Autodesk Inventor part; units mm, degrees
ref_plane "YZ Plane" through (0, 0, 0) normal (1, 0, 0) x (0, 1, 0)
ref_plane "XZ Plane" through (0, 0, 0) normal (0, 1, 0) x (-1, 0, 0)
ref_plane "XY Plane" through (0, 0, 0) normal (0, 0, 1) x (1, 0, 0)
sketch "Sketch1" plane through (0, 0, 0) normal (0, 0, 1) x (1, 0, 0)
  circle A0 centre (0, 0) radius 295
  circle A1 centre (0, 0) radius 168
  dimension "d0" = 590
  dimension "d1" = 336
extrude "Extrusion1" add sketch "Sketch1" along normal blind 100
sketch "Sketch2" plane through (0, 0, 100) normal (0, 0, 1) x (1, 0, 0)
  line L0 (-204.3933, 171.1712) -> (-160.5291, 171.1712) construction
  line L1 (-160.5291, 171.1712) -> (-160.5291, 111.0696) construction
  line L2 (-160.5291, 111.0696) -> (-204.3933, 111.0696) construction
  line L3 (-204.3933, 111.0696) -> (-204.3933, 171.1712) construction
  line L4 (-245.1262, 97.2034) -> (-201.262, 97.2034) construction
  line L5 (-201.262, 97.2034) -> (-201.262, 37.1018) construction
  line L6 (-201.262, 37.1018) -> (-245.1262, 37.1018) construction
  line L7 (-245.1262, 37.1018) -> (-245.1262, 97.2034) construction
  spline S0 degree 2 poles (-185.39, 119.3884) (-190.8195, 119.3884) (-198.437, 121.6574) (-201.8001, 123.2782) knots 0 0 0 1 2 2 2
  line L8 (-201.8001, 123.2782) -> (-201.8001, 131.625)
  line L9 (-201.8001, 131.625) -> (-201.3139, 131.625)
  spline S1 degree 2 poles (-201.3139, 131.625) (-198.0319, 128.5456) (-189.7255, 125.142) (-185.8763, 125.142) knots 0 0 0 1 2 2 2
  spline S2 degree 2 poles (-185.8763, 125.142) (-180.3657, 125.142) (-174.7336, 129.7206) (-174.7336, 133.4889) knots 0 0 0 1 2 2 2
  spline S3 degree 2 poles (-174.7336, 133.4889) (-174.7336, 136.4873) (-177.6915, 140.215) (-180.8925, 141.1469) knots 0 0 0 1 2 2 2
  spline S4 degree 2 poles (-180.8925, 141.1469) (-183.202, 141.7952) (-187.0513, 142.6866) (-189.9281, 143.4159) knots 0 0 0 1 2 2 2
  spline S5 degree 2 poles (-189.9281, 143.4159) (-192.5213, 144.1048) (-196.6137, 146.1712) (-198.1939, 147.8325) knots 0 0 0 1 2 2 2
  spline S6 degree 2 poles (-198.1939, 147.8325) (-199.7336, 149.4937) (-201.4354, 153.9508) (-201.4354, 156.8681) knots 0 0 0 1 2 2 2
  spline S7 degree 2 poles (-201.4354, 156.8681) (-201.4354, 162.9459) (-191.9541, 171.1712) (-184.6202, 171.1712) knots 0 0 0 1 2 2 2
  spline S8 degree 2 poles (-184.6202, 171.1712) (-180.4062, 171.1712) (-172.9508, 169.51) (-169.7498, 167.9297) knots 0 0 0 1 2 2 2
  line L10 (-169.7498, 167.9297) -> (-169.7498, 159.9881)
  line L11 (-169.7498, 159.9881) -> (-170.2361, 159.9881)
  spline S9 degree 2 poles (-170.2361, 159.9881) (-172.6267, 162.1761) (-180.0821, 165.4176) (-184.1745, 165.4176) knots 0 0 0 1 2 2 2
  spline S10 degree 2 poles (-184.1745, 165.4176) (-188.7936, 165.4176) (-194.5067, 161.0821) (-194.5067, 157.557) knots 0 0 0 1 2 2 2
  spline S11 degree 2 poles (-194.5067, 157.557) (-194.5067, 154.3965) (-191.1437, 150.6283) (-187.9832, 149.7774) knots 0 0 0 1 2 2 2
  spline S12 degree 2 poles (-187.9832, 149.7774) (-185.8763, 149.2101) (-179.758, 147.7514) (-177.732, 147.1437) knots 0 0 0 1 2 2 2
  spline S13 degree 2 poles (-177.732, 147.1437) (-172.5862, 145.5634) (-167.805, 139.202) (-167.805, 134.5424) knots 0 0 0 1 2 2 2
  spline S14 degree 2 poles (-167.805, 134.5424) (-167.805, 131.5845) (-170.1956, 125.9119) (-172.343, 123.9265) knots 0 0 0 1 2 2 2
  spline S15 degree 2 poles (-172.343, 123.9265) (-174.7336, 121.7385) (-180.8114, 119.3884) (-185.39, 119.3884) knots 0 0 0 1 2 2 2
  spline S16 degree 2 poles (-200.6367, 72.1629) (-200.6367, 65.3152) (-206.1877, 54.2942) (-210.8474, 51.2147) knots 0 0 0 1 2 2 2
  spline S17 degree 2 poles (-210.8474, 51.2147) (-214.6561, 48.8241) (-222.4762, 47.2034) (-228.554, 47.2034) knots 0 0 0 1 2 2 2
  line L12 (-228.554, 47.2034) -> (-240.0613, 47.2034)
  line L13 (-240.0613, 47.2034) -> (-240.0613, 97.2034)
  line L14 (-240.0613, 97.2034) -> (-228.6756, 97.2034)
  spline S18 degree 2 poles (-228.6756, 97.2034) (-221.6253, 97.2034) (-213.6027, 95.0964) (-210.7663, 93.2326) knots 0 0 0 1 2 2 2
  spline S19 degree 2 poles (-210.7663, 93.2326) (-205.9446, 90.0316) (-200.6367, 79.4562) (-200.6367, 72.1629) knots 0 0 0 1 2 2 2
  spline S20 degree 2 poles (-207.5654, 72.2439) (-207.5654, 77.9976) (-211.3741, 86.1418) (-215.1424, 88.4514) knots 0 0 0 1 2 2 2
  spline S21 degree 2 poles (-215.1424, 88.4514) (-217.8166, 90.0316) (-223.8539, 91.4498) (-228.3514, 91.4498) knots 0 0 0 1 2 2 2
  line L15 (-228.3514, 91.4498) -> (-233.4163, 91.4498)
  line L16 (-233.4163, 91.4498) -> (-233.4163, 52.957)
  line L17 (-233.4163, 52.957) -> (-228.3514, 52.957)
  spline S22 degree 2 poles (-228.3514, 52.957) (-223.9349, 52.957) (-217.2493, 54.3752) (-214.5346, 56.2796) knots 0 0 0 1 2 2 2
  spline S23 degree 2 poles (-214.5346, 56.2796) (-211.05, 58.6297) (-207.5654, 66.4092) (-207.5654, 72.2439) knots 0 0 0 1 2 2 2
  point P0 (0, 0)
extrude "Extrusion2" add sketch "Sketch2" along normal blind 20
sketch "Sketch3" plane through (0, 0, 100) normal (0, 0, 1) x (1, 0, 0)
  circle A0 centre (-107.4544, 206.725) radius 38.7006
  line L0 (0, 260.9541) -> (30, 208.9926)
  line L1 (0, 260.9541) -> (60, 260.9541) construction
  line L2 (30, 208.9926) -> (-30, 208.9926)
  line L3 (-30, 208.9926) -> (0, 260.9541)
  line L4 (74.2712, 223.542) -> (129.0294, 200.0839)
  line L5 (129.0294, 200.0839) -> (129.6987, 201.6462)
  line L6 (129.6987, 201.6462) -> (74.9405, 225.1043)
  line L7 (74.9405, 225.1043) -> (74.2712, 223.542)
  line L8 (74.2712, 223.542) -> (129.6987, 201.6462) construction
  line L9 (129.0294, 200.0839) -> (74.9405, 225.1043) construction
  line L10 (63.2876, 195.758) -> (118.0458, 172.2999)
  line L11 (118.0458, 172.2999) -> (118.7151, 173.8622)
  line L12 (118.7151, 173.8622) -> (63.9569, 197.3203)
  line L13 (63.9569, 197.3203) -> (63.2876, 195.758)
  line L14 (63.2876, 195.758) -> (118.7151, 173.8622) construction
  line L15 (118.0458, 172.2999) -> (63.9569, 197.3203) construction
  line L16 (86.0027, 247.306) -> (140.7609, 223.848)
  line L17 (140.7609, 223.848) -> (141.4302, 225.4103)
  line L18 (141.4302, 225.4103) -> (86.672, 248.8684)
  line L19 (86.672, 248.8684) -> (86.0027, 247.306)
  circle A1 centre (181.5681, 150.8575) radius 34.8144
  circle A2 centre (146.7537, 150.8575) radius 3.4311
  circle A3 centre (170.8099, 117.747) radius 3.4311
  circle A4 centre (209.7335, 130.3941) radius 3.4311
  circle A5 centre (209.7335, 171.3209) radius 3.4311
  circle A6 centre (170.8099, 183.9679) radius 3.4311
  circle A7 centre (222.3863, 63.4959) radius 44.0014
  line L20 (189.9505, 93.2287) -> (254.8222, 93.2287)
  line L21 (254.8222, 93.2287) -> (254.8222, 33.763)
  line L22 (254.8222, 33.763) -> (189.9505, 33.763)
  line L23 (189.9505, 33.763) -> (189.9505, 93.2287)
  line L24 (189.9505, 93.2287) -> (254.8222, 33.763) construction
  line L25 (254.8222, 93.2287) -> (189.9505, 33.763) construction
  point P0 (0, 0)
  point P1 (101.985, 212.5941)
  point P2 (91.0013, 184.8101)
  point P3 (189.9505, 93.2287)
  point P4 (189.9505, 93.2287)
  point P5 (254.8222, 93.2287)
  point P6 (254.8222, 93.2287)
  point P7 (189.9505, 33.763)
  point P8 (189.9505, 33.763)
  dimension "d6" = 60
  dimension "d7" = 60
  dimension "d8" = 60
  dimension "d9" = 60
  dimension "d12" = 360
extrude "Extrusion3" add sketch "Sketch3" along normal blind 20 contours A0 | L0 L2 L3 | L7 L6 L5 L4 | L13 L12 L11 L10 | L19 L18 L17 L16 | A5 A1 | A1 A5 | A4 A1 | A1 A4 | A6 A1 | A1 A6 | A3 A1 | A1 A3 | A2 A1 | A1 A2 | A7 L21 | L20 A7 | L21 L22 L23 L20 | A7 L22 | L23 A7
sketch "Sketch4" plane through (222.3863, 63.4959, 120) normal (0, 0, 1) x (1, 0, 0)
  line L0 (-27.8414, 23.9777) -> (27.8414, 23.9777)
  line L1 (27.8414, 23.9777) -> (27.8414, -23.9777)
  line L2 (27.8414, -23.9777) -> (-27.8414, -23.9777)
  line L3 (-27.8414, -23.9777) -> (-27.8414, 23.9777)
  line L4 (-27.8414, 23.9777) -> (27.8414, -23.9777) construction
  line L5 (27.8414, 23.9777) -> (-27.8414, -23.9777) construction
  point P0 (-222.3863, -63.4959)
  point P1 (0, 0)
extrude "Extrusion4" add sketch "Sketch4" along normal blind 10
properties part number "lab5CADfiguras"
The model under review builds one solid part; all positions refer to its coordinate system, in mm. A direction names the side the tool comes from. Coordinates: 2 decimals unless noted, no trailing zeros. Order: outer loops, then holes, each group sorted by start corner. A loop starts at its lowest first (then second) coordinate and runs counter-clockwise, first axis right, second up. Notation, with made-up numbers: (49, 20.25) -> (92, 20.25) arc R23 ccw to (92, 33.25) -> close; hole circle Ø8 at (56.5, 37.25). An arc over 180 degrees is marked (long way). Answer in a Markdown table with one row per item.
(1) Consider section A-A (y = 0). Write out the cut boundary in (x, z), plus the area to 3 significant figures.
Answers:
| item | result |
|---|---|
| outline | (-295, 0) -> (-168, 0) -> (-168, 100) -> (-295, 100) -> close; (168, 0) -> (295, 0) -> (295, 100) -> (168, 100) -> close |
| area | 25,400 mm² |
(2) Consider section B-B (x = -95.5). Write out the cut boundary in (y, z), plus the area to 3 significant figures.
Answers:
| item | result |
|---|---|
| outline | (-279.11, 0) -> (-138.22, 0) -> (-138.22, 100) -> (-279.11, 100) -> close; (138.22, 0) -> (279.11, 0) -> (279.11, 100) -> (243.53, 100) -> (243.53, 120) -> (169.92, 120) -> (169.92, 100) -> (138.22, 100) -> close |
| area | 29,700 mm² |
(3) Consider section D-D (y = -149). Write out the cut boundary in (x, z), plus the area to 3 significant figures.
Answers:
| item | result |
|---|---|
| outline | (-254.61, 0) -> (-77.61, 0) -> (-77.61, 100) -> (-254.61, 100) -> close; (77.61, 0) -> (254.61, 0) -> (254.61, 100) -> (77.61, 100) -> close |
| area | 35,400 mm² |
(4) Wall thickness on line 1 along Z through (x, y) = (-29.5, -201); line 2 along X through (y, z) = (41.5, 20); line 3 along Y through (x, z) = (0, 32): over which ranges is each line inside the solid? List them lowest first.
Answers:
| item | result |
|---|---|
| line 1 | 0 to 100 |
| line 2 | -292.07 to -162.79, 162.79 to 292.07 |
| line 3 | -295 to -168, 168 to 295 |
(5) The part is to be moulded in two halves that separate along Y. For faces 6 (the flat face through (114.434, 236.975, 109.86)), 7 (the flat face through (113, 235.74, 109.86)), 8 (the flat face through (-108, 207, 120)), say which applies: +Y half, -Y half, draft (parallel to the pull), parting line (faces both ways), or undercut.
Answers:
| item | result |
|---|---|
| face 6 | +Y half |
| face 7 | undercut |
| face 8 | draft |
(6) Consider section C-C (z = 14). Write out the cut boundary in (x, y), plus the area to 3 significant figures.
Answers:
| item | result |
|---|---|
| outline | circle Ø590 at (0, 0); hole circle Ø336 at (0, 0) |
| area | 185,000 mm² |
(7) Insertion check: pin 1 (10 mm diameter, centred on y = 68.5, z = 112, fed in from -X); pin 2 (6 mm diameter, centred on x = -237, z = 106.5, fed in from -Y); pin 3 (6 mm diameter, centred on x = 191.5, y = -4, fed in from +Z); pin 4 (1.5 mm diameter, centred on x = 151, z = 104, fed in from -Y). Each pin has a flat end and moves straight along its axis. Give the tip position at first contact, or say it passes through.
Answers:
| item | result |
|---|---|
| pin 1 | x = -240.06 |
| pin 2 | y = 47.2 |
| pin 3 | z = 100 |
| pin 4 | through |
(8) Machinability: for faces 1 (the cylindrical face through (-63.95, 287.985, 49.3)), 2 (the flat face through (-185, 146, 120)), 3 (the flat face through (0, 208.993, 110)), 4 (the flat face through (-15.21, 234.61, 109.86)), 5 (the cylindrical face through (-138.17, 230.27, 109.86)), which of the approach directions +Z, -Z, +X, -X, +Y, -Y give a long, thin tool a straight path to every point of the face, cutting with its end or side? Answer none if there is none.
Answers:
| item | result |
|---|---|
| face 1 | +Z, -Z |
| face 2 | +Z, +X, -X, +Y, -Y |
| face 3 | +Z, -Y |
| face 4 | +Z, +Y |
| face 5 | +Z |
